For this review, take the finished solid that the model builds, in its own axes (mm). Face numbers are marked on the shaded views. Round coordinates to 2 decimals unless told otherwise and drop trailing zeros. Write each loop counter-clockwise with the first axis right and the second up, starting at its lowest first coordinate (ties: lowest second). Pieces come first, ordered by that corner, then holes. Notation, with made-up numbers: M 85.5,16.5 L 100.5,16.5 A22 cw 100.5,44.5 Z; hole C 17,-31.5 d9. An arc over 180 degrees is marked long. Use one line per item in the form item = value. Start each with the question number.
Item 1: Add section A-A (z = 5.5). State the section outline as (x, y) points (3 decimals).
Item 2: Add section C-C (x = 27.5). State the section outline as (y, z) points, and give its area (3 significant figures).
Item 3: For line 1 (Z direction, x = -15.5, y = 25.5); line 2 (X direction, y = 33.5, z = 3.75); line 3 (Y direction, x = 24.5, z = 11.5), list the stretches that pass through material, from the lowest coordinate up. Write a range as [from, to].
Item 4: For P1, Ø6, axis at y = 60, z = 11.5, coming from the +X side; P2, Ø8, axis at x = -19.5, y = 61.5, coming from the -Z side; P3, Ø4, axis at x = -4, z = 9, coming from the -Y side, all flat-tipped, find the tip position at first contact; note any pin that passes through.
Item 5: Draft analysis for pull direction X (two halves, no side actions). For the marked faces 1, 2 and 3, state which applies: released by +X, released by -X, zero draft, split by the parting line, or undercut.
Item 6: Add section B-B (z = -3.75). State the section outline as (x, y) points.
Item 7: Add section D-D (y = 57). State the section outline as (x, z) points, and give its area (3 significant figures).
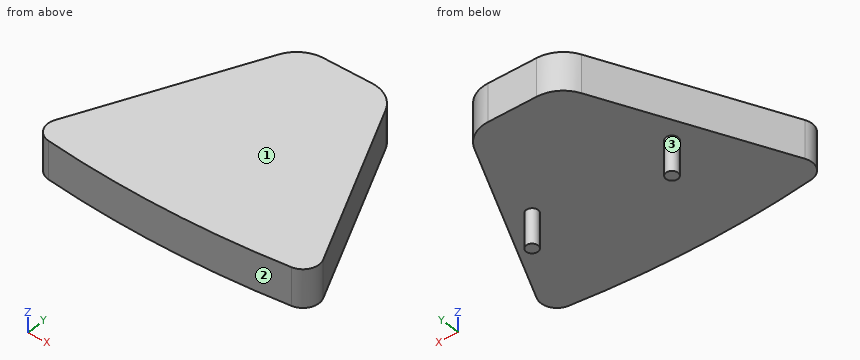
from build123d import *

# Parameters (mm, degrees)
BOSS_EXTRUDE1_DEPTH = 15
SKETCH2_R           = 2.38125
BOSS_EXTRUDE2_DEPTH = 13.716


with BuildPart() as part:
    # Sketch1 → Boss-Extrude1 (new body)
    with BuildSketch(Plane.XY):
        with BuildLine():
            Line((-52.739408914, 11.9161458), (-21.023817827, 79.5593995))
            ThreePointArc((-21.023817827, 79.5593995), (-16.337460141, 84.886226851), (-9.525, 86.868))
            Line((-9.525, 86.868), (9.525, 86.868))
            ThreePointArc((9.525, 86.868), (16.337460141, 84.886226851), (21.023817827, 79.5593995))
            Line((21.023817827, 79.5593995), (52.739408914, 11.9161458))
            ThreePointArc((52.739408914, 11.9161458), (52.54682937, 6.1473129), (47.762912079, 2.917660402))
            ThreePointArc((47.762912079, 2.917660402), (0, 0), (-47.762912079, 2.917660402))
            ThreePointArc((-47.762912079, 2.917660402), (-52.54682937, 6.1473129), (-52.739408914, 11.9161458))
        make_face()
    extrude(amount=BOSS_EXTRUDE1_DEPTH)

    # Sketch2 → Boss-Extrude2 (add)
    with BuildSketch(Plane(origin=(0, 0, 0), x_dir=(-1, 0, 0), z_dir=(0, 0, -1))):
        with Locations((-27.5, 44.45)):
            Circle(SKETCH2_R)
        with Locations((27.5, 44.45)):
            Circle(SKETCH2_R)
    extrude(amount=BOSS_EXTRUDE2_DEPTH)


solid = part.part
Calculated:
q1.outline = M -52.739,11.916 A6.35 ccw -47.763,2.918 A392.405 ccw 47.763,2.918 A6.35 ccw 52.739,11.916 L 21.024,79.559 A12.7 ccw 9.525,86.868 L -9.525,86.868 A12.7 ccw -21.024,79.559 Z
q2.outline = M 0.96,0 L 42.07,0 L 42.07,-13.72 L 46.83,-13.72 L 46.83,0 L 65.75,0 L 65.75,15 L 0.96,15 Z
q2.area = 1,040 mm^2
q3.line_1 = [0, 15]
q3.line_2 = [-42.62, 42.62]
q3.line_3 = [0.77, 72.15]
q4.P1 = 31.6
q4.P2 = 0
q4.P3 = 0.01
q5.face_1 = zero draft
q5.face_2 = split by the parting line
q5.face_3 = undercut
q6.outline = C -27.5,44.45 d4.76; C 27.5,44.45 d4.76
q7.outline = M -31.6,0 L 31.6,0 L 31.6,15 L -31.6,15 Z
q7.area = 948 mm^2
